Source: CAD feature listing. Evaluate the final solid. Frame: model axes, mm. A direction names the side the tool comes from. Give positions to 0.01 mm unless a question says otherwise; leave off trailing zeros. Write each loop counter-clockwise with the first axis right and the second up, starting at its lowest first coordinate (ties: lowest second). Pieces come first, ordered by that corner, then holes. Notation, with made-up numbers: M 72.25,10.5 L 77.25,10.5 A15 cw 77.25,30.5 Z; hole C 23.25,12 d5. An arc over 180 degrees is marked long. Return JSON: item names as keys, results as strings.
```python
from build123d import *

# Parameters (mm, degrees)
PAD_DEPTH       = 73
POCKET_DEPTH    = 17.001
SKETCH006_R     = 1.4
POCKET001_DEPTH = 5.7
POCKET002_DEPTH = 2.5
POCKET003_DEPTH = 2
SKETCH007_R     = 1.65
POCKET004_DEPTH = 17.001
POCKET007_DEPTH = 1.5
SKETCH021_R     = 1.15
POCKET012_DEPTH = 5.7
POCKET014_DEPTH = 1.8
POCKET015_DEPTH = 2.3
POCKET017_DEPTH = 17.001
SKETCH028_W     = 44
SKETCH028_H     = 65
POCKET018_DEPTH = 8.2


with BuildPart() as part:
    # Sketch → Pad (new body)
    with BuildSketch(Plane.XZ):
        with BuildLine():
            Line((-44, 0), (-34, 0))
            Line((-34, 0), (-34, 12))
            ThreePointArc((-32, 14), (-33.414214, 13.414214), (-34, 12))
            Line((-32, 14), (32, 14))
            ThreePointArc((34, 12), (33.414214, 13.414214), (32, 14))
            Line((34, 0), (34, 12))
            Line((34, 0), (44, 0))
            Line((44, 0), (44, 6.7))
            ThreePointArc((44, 6.7), (43.707107, 7.407107), (43, 7.7))
            Line((43, 7.7), (37, 7.7))
            ThreePointArc((36, 8.7), (36.292893, 7.992893), (37, 7.7))
            Line((36, 8.7), (36, 8.9))
            ThreePointArc((37, 9.9), (36.292893, 9.607107), (36, 8.9))
            Line((37, 9.9), (43, 9.9))
            ThreePointArc((43, 9.9), (43.707107, 10.192893), (44, 10.9))
            Line((44, 17), (44, 10.9))
            Line((-44, 17), (44, 17))
            Line((-44, 10.9), (-44, 17))
            ThreePointArc((-44, 10.9), (-43.707107, 10.192893), (-43, 9.9))
            Line((-37, 9.9), (-43, 9.9))
            ThreePointArc((-36, 8.9), (-36.292893, 9.607107), (-37, 9.9))
            Line((-36, 8.7), (-36, 8.9))
            ThreePointArc((-37, 7.7), (-36.292893, 7.992893), (-36, 8.7))
            Line((-43, 7.7), (-37, 7.7))
            ThreePointArc((-43, 7.7), (-43.707107, 7.407107), (-44, 6.7))
            Line((-44, 0), (-44, 6.7))
        make_face()
    extrude(amount=-PAD_DEPTH)

    # Sketch001 → Pocket (cut, through all)
    with BuildSketch(Plane.XY):
        Polygon((-66, 80), (-36, 50), (-36, 20), (-66, -10), align=None)
        Polygon((36, 20), (66, -10), (66, 80), (36, 50), align=None)
    extrude(amount=POCKET_DEPTH, mode=Mode.SUBTRACT)

    # Sketch006 → Pocket001 (cut)
    with BuildSketch(Plane.XY):
        with Locations((-40, 60)):
            Circle(SKETCH006_R)
        with Locations((40, 60)):
            Circle(SKETCH006_R)
        with Locations((40, 5)):
            Circle(SKETCH006_R)
        with Locations((-40, 5)):
            Circle(SKETCH006_R)
    extrude(amount=POCKET001_DEPTH, mode=Mode.SUBTRACT)

    # Sketch005 (on DatumPlane) → Pocket002 (cut)
    with BuildSketch(Plane.XY.offset(3.6)):
        Polygon((-37.4, 3.498889), (-37.4, 6.501111), (-40, 8.002221), (-42.6, 6.501111), (-42.6, 3.498889), (-42.6, -6.501111), (-37.4, -6.501111), align=None)
        Polygon((42.6, 3.498889), (42.6, 6.501111), (40, 8.002221), (37.4, 6.501111), (37.4, 3.498889), (37.4, -6.501111), (42.6, -6.501111), align=None)
        Polygon((-40, 56.997779), (-37.4, 58.498889), (-37.4, 61.501111), (-37.4, 71.501111), (-42.6, 71.501111), (-42.6, 61.501111), (-42.6, 58.498889), align=None)
        Polygon((37.4, 58.498889), (40, 56.997779), (42.6, 58.498889), (42.6, 61.501111), (42.6, 71.501111), (37.4, 71.501111), (37.4, 61.501111), align=None)
    extrude(amount=POCKET002_DEPTH, mode=Mode.SUBTRACT)

    # Sketch004 (on DatumPlane) → Pocket003 (cut)
    with BuildSketch(Plane.XY.offset(1.6)):
        Polygon((-40, 1.997779), (-37.4, 3.498889), (-37.4, 6.501111), (-40, 8.002221), (-42.6, 6.501111), (-42.6, 3.498889), align=None)
        Polygon((40, 1.997779), (42.6, 3.498889), (42.6, 6.501111), (40, 8.002221), (37.4, 6.501111), (37.4, 3.498889), align=None)
        Polygon((40, 56.997779), (42.6, 58.498889), (42.6, 61.501111), (40, 63.002221), (37.4, 61.501111), (37.4, 58.498889), align=None)
        Polygon((-40, 56.997779), (-37.4, 58.498889), (-37.4, 61.501111), (-40, 63.002221), (-42.6, 61.501111), (-42.6, 58.498889), align=None)
    extrude(amount=POCKET003_DEPTH, mode=Mode.SUBTRACT)

    # Sketch007 → Pocket004 (cut, through all)
    with BuildSketch(Plane.XY):
        with Locations((-16, 40.1)):
            Circle(SKETCH007_R)
        with Locations((-16, 25.9)):
            Circle(SKETCH007_R)
        with Locations((16, 40.1)):
            Circle(SKETCH007_R)
        with Locations((16, 25.9)):
            Circle(SKETCH007_R)
    extrude(amount=POCKET004_DEPTH, mode=Mode.SUBTRACT)

    # Sketch008 (on DatumPlane) → Pocket007 (cut)
    with BuildSketch(Plane.XY.offset(17)):
        Polygon((-18.9, 41.774316), (-18.9, 38.425684), (-16, 36.751368), (-13.1, 38.425684), (-13.1, 41.774316), (-16, 43.448632), align=None)
        Polygon((13.1, 41.774316), (13.1, 38.425684), (16, 36.751368), (18.9, 38.425684), (18.9, 41.774316), (16, 43.448632), align=None)
        Polygon((-18.9, 27.574316), (-18.9, 24.225684), (-16, 22.551368), (-13.1, 24.225684), (-13.1, 27.574316), (-16, 29.248632), align=None)
        Polygon((13.1, 27.574316), (13.1, 24.225684), (16, 22.551368), (18.9, 24.225684), (18.9, 27.574316), (16, 29.248632), align=None)
    extrude(amount=-POCKET007_DEPTH, mode=Mode.SUBTRACT)

    # Sketch021 (on DatumPlane) → Pocket012 (cut)
    with BuildSketch(Plane.XY.offset(17)):
        with Locations((-2.7, 68.5)):
            Circle(SKETCH021_R)
        with Locations((2.7, 68.5)):
            Circle(SKETCH021_R)
        with Locations((-40, 5)):
            Circle(SKETCH021_R)
        with Locations((40, 5)):
            Circle(SKETCH021_R)
    extrude(amount=-POCKET012_DEPTH, mode=Mode.SUBTRACT)

    # Sketch024 (on DatumPlane) → Pocket014 (cut)
    with BuildSketch(Plane.XY.offset(13.1)):
        Polygon((0.6, 67.287564), (2.7, 66.075129), (4.8, 67.287564), (4.8, 69.712436), (2.7, 70.924871), (0.6, 69.712436), align=None)
        Polygon((40, 7.424871), (37.9, 6.212436), (37.9, 3.787564), (40, 2.575129), (42.1, 3.787564), (42.1, 6.212436), align=None)
        Polygon((-37.9, 6.212436), (-40, 7.424871), (-42.1, 6.212436), (-42.1, 3.787564), (-40, 2.575129), (-37.9, 3.787564), align=None)
        Polygon((-4.8, 67.287564), (-2.7, 66.075129), (-0.6, 67.287564), (-0.6, 69.712436), (-2.7, 70.924871), (-4.8, 69.712436), align=None)
    extrude(amount=-POCKET014_DEPTH, mode=Mode.SUBTRACT)

    # Sketch025 (on DatumPlane) → Pocket015 (cut)
    with BuildSketch(Plane.XY.offset(13.1)):
        Polygon((2.7, 66.075129), (4.8, 67.287564), (4.8, 69.712436), (4.8, 89.712436), (0.6, 89.712436), (0.6, 69.712436), (0.6, 67.287564), align=None)
        Polygon((40, 7.424871), (37.9, 6.212436), (37.9, 3.787564), (37.9, -16.212436), (42.1, -16.212436), (42.1, 3.787564), (42.1, 6.212436), align=None)
        Polygon((-40, 7.424871), (-42.1, 6.212436), (-42.1, 3.787564), (-42.1, -16.212436), (-37.9, -16.212436), (-37.9, 3.787564), (-37.9, 6.212436), align=None)
        Polygon((-2.7, 66.075129), (-0.6, 67.287564), (-0.6, 69.712436), (-0.6, 89.712436), (-4.8, 89.712436), (-4.8, 69.712436), (-4.8, 67.287564), align=None)
    extrude(amount=POCKET015_DEPTH, mode=Mode.SUBTRACT)

    # Sketch027 → Pocket017 (cut, through all)
    with BuildSketch(Plane.XY):
        with BuildLine():
            Line((-65, 65), (-15.656854, 65))
            ThreePointArc((-15.656854, 65), (-14.891487, 65.152241), (-14.242641, 65.585786))
            Line((-14.242641, 65.585786), (-7.414214, 72.414214))
            ThreePointArc((-6, 73), (-6.765367, 72.847759), (-7.414214, 72.414214))
            Line((-6, 73), (6, 73))
            ThreePointArc((7.414214, 72.414214), (6.765367, 72.847759), (6, 73))
            Line((14.242641, 65.585786), (7.414214, 72.414214))
            ThreePointArc((14.242641, 65.585786), (14.891487, 65.152241), (15.656854, 65))
            Line((15.656854, 65), (65, 65))
            Line((65, 65), (65, 97))
            Line((65, 97), (-65, 97))
            Line((-65, 65), (-65, 97))
        make_face()
    extrude(amount=POCKET017_DEPTH, mode=Mode.SUBTRACT)

    # Sketch028 (on DatumPlane) → Pocket018 (cut)
    with BuildSketch(Plane.XY.offset(17)):
        with Locations((-58, 65)):
            Rectangle(SKETCH028_W, SKETCH028_H)
        with Locations((58, 65)):
            Rectangle(SKETCH028_W, SKETCH028_H)
    extrude(amount=-POCKET018_DEPTH, mode=Mode.SUBTRACT)


solid = part.part
```
1) Cut plane B-B, the plane y = 44.5. Return the cut outline in (x, z), then the cut area to 3 significant figures.
Numbers:
{"outline": "M -36,0 L -34,0 L -34,12 A2 cw -32,14 L 32,14 A2 cw 34,12 L 34,0 L 36,0 L 36,17 L -36,17 Z", "area": "274 mm²"}
2) Set-up query: faces 1 (the face through (33.43, 32.04, 13.4)), 2 (the face through (-3, 70, 15.4)), 3 (the face through (40, 1, 3.6)), 4 (the face through (-38.718, 57.738, 3.818)). Return all of +Z, -Z, +X, -X, +Y, -Y with unobstructed straight access to the full face (end or side cutting, diameter ignored); none if empty.
Numbers:
{"face 1": "-Z, +Y, -Y", "face 2": "-Z, +Y", "face 3": "-Y", "face 4": "none"}
3) Cut plane A-A, the plane y = 25.9. Return the cut outline in (x, z), then the cut area to 3 significant figures.
Numbers:
{"outline": "M -36,0 L -34,0 L -34,12 A2 cw -32,14 L -17.65,14 L -17.65,15.5 L -18.9,15.5 L -18.9,17 L -36,17 Z; M -14.35,14 L 14.35,14 L 14.35,15.5 L 13.1,15.5 L 13.1,17 L -13.1,17 L -13.1,15.5 L -14.35,15.5 Z; M 17.65,14 L 32,14 A2 cw 34,12 L 34,0 L 36,0 L 36,17 L 18.9,17 L 18.9,15.5 L 17.65,15.5 Z", "area": "246 mm²"}
4) Contact query for flat-ended pins moving along their axis: pin 1 Ø1.2 at (y, z) = (26, 16) entering from -X; pin 2 Ø6 at (x, y) = (3.5, 12) entering from -Z; pin 3 Ø2 at (y, z) = (41, 3.5) entering from +X; pin 4 Ø2 at (x, y) = (16, 40.1) entering from +Z. Output: stop coordinate, or through.
Numbers:
{"pin 1": "stops at x = -36", "pin 2": "stops at z = 14", "pin 3": "stops at x = 36", "pin 4": "passes through"}
5) Draft query along X for faces 5 (the face through (-40, 16, 14)), 6 (the face through (-40, 7, 7.7)), 7 (the face through (-2.08, 69.47, 16.21)). Return one class per face: released by +X, released by -X, zero draft, split by the parting line, or undercut.
Numbers:
{"face 5": "released by -X", "face 6": "zero draft", "face 7": "undercut"}
6) Cut plane C-C, the plane x = 35. Return the cut outline in (y, z).
Numbers:
{"outline": "M 0,0 L 65,0 L 65,17 L 0,17 Z"}
7) Line query: line 1 (X direction, y = 60, z = 1); line 2 (Y direction, x = 16, z = 14.55); line 3 (X direction, y = 36, z = 6.5). Output: solid intervals per line, ascending. Write a range as [from, to].
Numbers:
{"line 1": "x = [-44, -41.4], [-38.6, -34], [34, 38.6], [41.4, 44]", "line 2": "y = [0, 24.25], [27.55, 38.45], [41.75, 65]", "line 3": "x = [-36, -34], [34, 36]"}
8) Cut plane D-D, the plane y = 68.5. Return the cut outline in (x, z).
Numbers:
{"outline": "M -11.33,14 L -4.8,14 L -4.8,15.4 L -3.85,15.4 L -3.85,17 L -11.33,17 Z; M -1.55,15.4 L -0.6,15.4 L -0.6,14 L 0.6,14 L 0.6,15.4 L 1.55,15.4 L 1.55,17 L -1.55,17 Z; M 3.85,15.4 L 4.8,15.4 L 4.8,14 L 11.33,14 L 11.33,17 L 3.85,17 Z"}
